Here's how the part is built. I have some questions about the finished solid (model axes, mm). A direction names the side the tool comes from. Give positions to 0.01 mm unless a question says otherwise; leave off trailing zeros. Write each loop counter-clockwise with the first axis right and the second up, starting at its lowest first coordinate (ties: lowest second). Pieces come first, ordered by that corner, then holes. Notation, with made-up numbers: (71.5, 1) -> (80.5, 1) arc R18 cw to (80.5, 12) -> close; hole circle Ø7 at (-0.75, -1.5). An arc over 180 degrees is marked (long way). Return JSON: item names as keys, results as strings.
from build123d import *

# Parameters (mm, degrees)
SKETCH1_R           = 38.1
BOSS_EXTRUDE1_DEPTH = 5.588
SKETCH5_R           = 38.1
SKETCH5_R_2         = 31.75
BOSS_EXTRUDE3_DEPTH = 16.764
CUT_EXTRUDE2_START  = -5.588
CUT_EXTRUDE2_DEPTH  = 5.588
BOSS_EXTRUDE4_START = -5.588
BOSS_EXTRUDE4_DEPTH = 5.588
CIRPATTERN1_COUNT   = 8


with BuildPart() as part:
    # Sketch1 → Boss-Extrude1 (new body)
    with BuildSketch(Plane(origin=(0, 0, 0), x_dir=(1, 0, 0), z_dir=(0, 1, 0))):
        with Locations(Location((0, 0, 0), (0, 0, 270))):
            Circle(SKETCH1_R)
    extrude(amount=BOSS_EXTRUDE1_DEPTH)

    # Sketch5 → Boss-Extrude3 (add)
    with BuildSketch(Plane(origin=(0, 5.588, 0), x_dir=(1, 0, 0), z_dir=(0, 1, 0))):
        with Locations(Location((0, 0, 0), (0, 0, 270))):
            Circle(SKETCH5_R)
        with Locations(Location((0, 0, 0), (0, 0, 270))):
            Circle(SKETCH5_R_2, mode=Mode.SUBTRACT)
    extrude(amount=BOSS_EXTRUDE3_DEPTH)

    # Sketch6 → Cut-Extrude2 (cut)
    with BuildSketch(Plane(origin=(0, 22.352, 0), x_dir=(1, 0, 0), z_dir=(0, 1, 0)).offset(CUT_EXTRUDE2_START)):
        with BuildLine():
            Line((-1.524, -32.452967385), (-1.524, -36.793402908))
            Line((-1.524, -36.793402908), (1.524, -36.793402908))
            Line((1.524, -36.793402908), (1.524, -32.452967385))
            Line((1.524, -32.452967385), (1.907415329, -32.452967385))
            Line((1.907415329, -32.452967385), (1.907415329, -31.817967385))
            Line((1.907415329, -31.817967385), (0.393317037, -31.817967385))
            Line((0.393317037, -31.817967385), (0.393317037, -31.747563713))
            ThreePointArc((0.393317037, -31.747563713), (0, -31.75), (-0.393317037, -31.747563713))
            Line((-0.393317037, -31.747563713), (-0.393317037, -31.817967385))
            Line((-0.393317037, -31.817967385), (-1.907415329, -31.817967385))
            Line((-1.907415329, -31.817967385), (-1.907415329, -32.452967385))
            Line((-1.907415329, -32.452967385), (-1.524, -32.452967385))
        make_face()
    cut_extrude2 = extrude(amount=CUT_EXTRUDE2_DEPTH, mode=Mode.SUBTRACT)

    # Sketch6_4 → Boss-Extrude4 (add)
    with BuildSketch(Plane(origin=(0, 22.352, 0), x_dir=(1, 0, 0), z_dir=(0, 1, 0)).offset(BOSS_EXTRUDE4_START)):
        with BuildLine():
            ThreePointArc((-3.407999769, -31.566565185), (-2.467092572, -31.654003763), (-1.524, -31.713402908))
            ThreePointArc((-1.524, -31.713402908), (-0.958810667, -31.735519251), (-0.393317037, -31.747563713))
            Line((-0.393317037, -31.747563713), (-0.393317037, -29.857063133))
            ThreePointArc((-0.393317037, -29.857063133), (-2.08401096, -30.388474513), (-3.407999769, -31.566565185))
        make_face()
        with BuildLine():
            ThreePointArc((0.393317037, -31.747563713), (0.958810667, -31.735519251), (1.524, -31.713402908))
            ThreePointArc((1.524, -31.713402908), (2.467092572, -31.654003763), (3.407999769, -31.566565185))
            ThreePointArc((3.407999769, -31.566565185), (2.08401096, -30.388474513), (0.393317037, -29.857063133))
            Line((0.393317037, -29.857063133), (0.393317037, -31.747563713))
        make_face()
    boss_extrude4 = extrude(amount=BOSS_EXTRUDE4_DEPTH)

    # CirPattern1: Cut-Extrude2, Boss-Extrude4 ×8 about axis
    cirpattern1_axis = Axis((0, 0, 0), (0, 1, 0))
    add([cut_extrude2.rotate(cirpattern1_axis, i * 360 / CIRPATTERN1_COUNT) for i in range(1, CIRPATTERN1_COUNT)], mode=Mode.SUBTRACT)
    add([boss_extrude4.rotate(cirpattern1_axis, i * 360 / CIRPATTERN1_COUNT) for i in range(1, CIRPATTERN1_COUNT)])


solid = part.part
1. Suppose I cut it at B-B, the plane z = 13.5. List the corners of the cut face in (x, y) for me.
Taken from the geometry:
{"outline": "(-35.63, 0) -> (35.63, 0) -> (35.63, 22.35) -> (28.74, 22.35) -> (28.74, 5.59) -> (-28.74, 5.59) -> (-28.74, 22.35) -> (-35.63, 22.35) -> close"}
2. For pin 1 Ø4 at (x, y) = (27, 9) entering from +Z; pin 2 Ø2 at (y, z) = (19.5, -14.5) entering from +X; pin 3 Ø4 at (x, y) = (14.5, 19) entering from -Z, each with a flat end and sliding along its axis, tell me the tip position at first contact or that it passes through.
Taken from the geometry:
{"pin 1": "stops at z = 28.75", "pin 2": "stops at x = 35.63", "pin 3": "stops at z = -35.99"}
3. Suppose I cut it at A-A, the plane y = 15. List the corners of the cut face in (x, z) for me, and give its area (3 significant figures).
Taken from the geometry:
{"outline": "circle Ø76.2 at (0, 0); hole circle Ø63.5 at (0, 0)", "area": "1,390 mm²"}
4. If I drill on line 1 (X direction, y = 9.25, z = 0); line 2 (X direction, y = 18.75, z = 0); line 3 (Y direction, x = 19.5, z = 18), over which ranges is the centre line in solid material (lowest first)? Write a range as [from, to].
Taken from the geometry:
{"line 1": "x = [-38.1, -31.75], [31.75, 38.1]", "line 2": "x = [-38.1, -36.79], [36.79, 38.1]", "line 3": "y = [0, 5.59]"}
5. Suppose I cut it at C-C, the plane z = -5.5. List the corners of the cut face in (x, y) for me.
Taken from the geometry:
{"outline": "(-37.7, 0) -> (37.7, 0) -> (37.7, 22.35) -> (31.27, 22.35) -> (31.27, 5.59) -> (-31.27, 5.59) -> (-31.27, 22.35) -> (-37.7, 22.35) -> close"}
6. Which directions (+Z, -Z, +X, -X, +Y, -Y) give clear straight access to the entire face, cutting with the end or side of a thin tool? Please do faces 5 (the face through (31, 16.764, 2)), 6 (the face through (23.383, 19.519, 25.538)).
Taken from the geometry:
{"face 5": "none", "face 6": "+Y"}
7. If we mould it in two halves opening along Y, with no side actions, what happens to faces 1 (the face through (24, 16.764, 24)), 2 (the face through (23, 16.764, 21)), 3 (the face through (-2, 16.764, 31)), 4 (the face through (-25.581, 19.519, -23.426))? For each: released by +Y, released by -Y, zero draft, split by the parting line, or undercut.
Taken from the geometry:
{"face 1": "released by +Y", "face 2": "undercut", "face 3": "undercut", "face 4": "zero draft"}
